For this review, take the finished solid that the model builds, in its own axes (mm). Face numbers are marked on the shaded views. A direction names the side the tool comes from. Round coordinates to 2 decimals unless told otherwise and drop trailing zeros. Order: outer loops, then holes, each group sorted by start corner. A loop starts at its lowest first (then second) coordinate and runs counter-clockwise, first axis right, second up. Notation, with made-up numbers: (84, -14) -> (103, -14) arc R15 ccw to (103, 11) -> close; hole circle Ø8 at (68, 85). An arc over 180 degrees is marked (long way). Put each result on its own line as item: value. Start each with the question number.
```python
from build123d import *

# Parameters (mm, degrees)
F0_W     = 133
F0_H     = 1800
F2_DEPTH = 12
F3_W     = 133
F3_H     = 12
F3_W_2   = 12
F3_H_2   = 188
F4_DEPTH = 630
F5_DEPTH = 1800.001
F6_START = 400
F1_W     = 50
F1_H     = 12
F6_DEPTH = 1400


with BuildPart() as f2:
    # F0 (on Front) → F2 (new body)
    with BuildSketch(Plane.XZ):
        with Locations((-66.5, 900)):
            Rectangle(F0_W, F0_H)
        with BuildLine():
            Line((-30, 1150), (-103, 1150))
            ThreePointArc((-103, 1150), (-110.0710678119, 1152.9289321881), (-113, 1160))
            Line((-113, 1160), (-113, 1240))
            ThreePointArc((-113, 1240), (-110.0710678119, 1247.0710678119), (-103, 1250))
            Line((-103, 1250), (-30, 1250))
            ThreePointArc((-30, 1250), (-22.9289321881, 1247.0710678119), (-20, 1240))
            Line((-20, 1240), (-20, 1160))
            ThreePointArc((-20, 1160), (-22.9289321881, 1152.9289321881), (-30, 1150))
        make_face(mode=Mode.SUBTRACT)
    extrude(amount=-F2_DEPTH)

    # F3 (on face) → F4 (join)
    with BuildSketch(Plane.XZ):
        with Locations((-66.5, 406)):
            Rectangle(F3_W, F3_H)
        with Locations((-66.5, 856)):
            Rectangle(F3_W, F3_H)
        with Locations((-66.5, 706)):
            Rectangle(F3_W, F3_H)
        with Locations((-66.5, 1006)):
            Rectangle(F3_W, F3_H)
        with Locations((-6, 1206)):
            Rectangle(F3_W_2, F3_H_2)
        Polygon((-12, 1300), (0, 1300), (0, 1312), (-133, 1312), (-133, 1300), align=None)
        Polygon((0, 1100), (0, 1112), (-12, 1112), (-133, 1112), (-133, 1100), align=None)
        with Locations((-66.5, 1456)):
            Rectangle(F3_W, F3_H)
        with Locations((-66.5, 1606)):
            Rectangle(F3_W, F3_H)
        with Locations((-66.5, 1794)):
            Rectangle(F3_W, F3_H)
    extrude(amount=F4_DEPTH)

    # F1 (on Top) → F5 (cut, through all)
    with BuildSketch(Plane.XY):
        Polygon((-50, -630), (-133, 0), (-133, -630), align=None)
    extrude(amount=F5_DEPTH, mode=Mode.SUBTRACT)

    # F1 (on Top) → F6 (join)
    with BuildSketch(Plane.XY.offset(F6_START)):
        with Locations((-25, -636)):
            Rectangle(F1_W, F1_H)
    extrude(amount=F6_DEPTH)


with BuildPart() as f7_1:
    # F7: copy of F2
    add(f2.part)


solid = f2.part
```
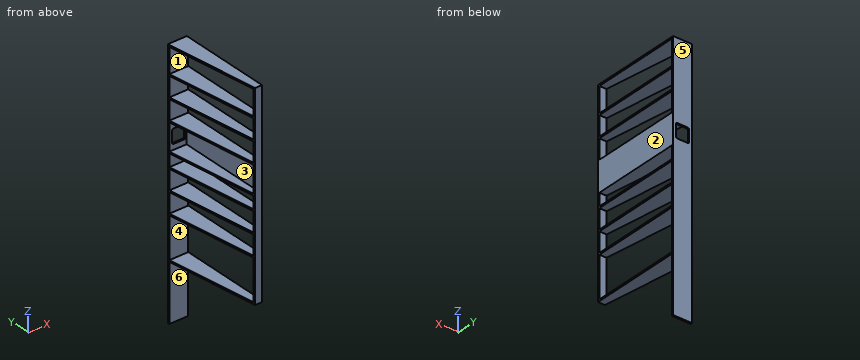
Item 1: Mouldability with a two-part tool opening along Y and no side actions: class the marked faces 4, 5 and 6 as +Y half, -Y half, draft (parallel to the pull), parting line (faces both ways), or undercut.
Item 2: For L1, parallel to Y at x = -14.5, z = 946; L2, parallel to Y at x = -8, z = 388.5; L3, parallel to X at y = -491, z = 1106, list the stretches that pass through material, from the lowest coordinate up.
Item 3: Insertion check: pin 1 Ø13 at (y, z) = (-635.5, 803) entering from -X; pin 2 Ø1.5 at (x, z) = (-78.5, 289) entering from -Y; pin 3 Ø1.5 at (x, y) = (-59.5, -272) entering from -Z. Each pin has a flat end and moves straight along its axis. Give the tip position at first contact, or say it passes through.
Item 4: Consider section D-D, the plane z = 275. Write out the cut boundary in (x, y), plus the area to 3 significant figures.
Item 5: Consider section B-B, the plane z = 1267.5. Write out the cut boundary in (x, y).
Item 6: Consider section A-A, the plane z = 1041. Write out the cut boundary in (x, y), plus the area to 3 significant figures.
Item 7: Consider section C-C, the plane y = -431. Count the separate pieces of the cut face and the enclosed holes in it, plus the area to 3 significant figures.
Item 8: Tool access review of the marked faces 1, 2 and 3: name each direction out of +Z, -Z, +X, -X, +Y, -Y from which nothing blocks a thin tool from reaching the whole face with its end or side.
Evaluation:
1. face 4: undercut
1. face 5: +Y half
1. face 6: -Y half
2. L1: y = -642 to -630, 0 to 12
2. L2: y = 0 to 12
2. L3: x = -68.31 to 0
3. pin 1: stops at x = -50
3. pin 2: stops at y = 0
3. pin 3: stops at z = 400
4. outline: (-133, 0) -> (0, 0) -> (0, 12) -> (-133, 12) -> close
4. area: 1,600 mm^2
5. outline: (-133, 0) -> (-12, 0) -> (-12, -630) -> (-50, -630) -> (-50, -642) -> (0, -642) -> (0, 12) -> (-133, 12) -> close
6. outline: (-133, 0) -> (0, 0) -> (0, 12) -> (-133, 12) -> close; (-50, -642) -> (0, -642) -> (0, -630) -> (-50, -630) -> close
6. area: 2,200 mm^2
7. separate pieces: 8
7. enclosed holes: 0
7. area: 10,500 mm^2
8. face 1: +X, -X
8. face 2: +Z, -Z, +X, +Y, -Y
8. face 3: -X
